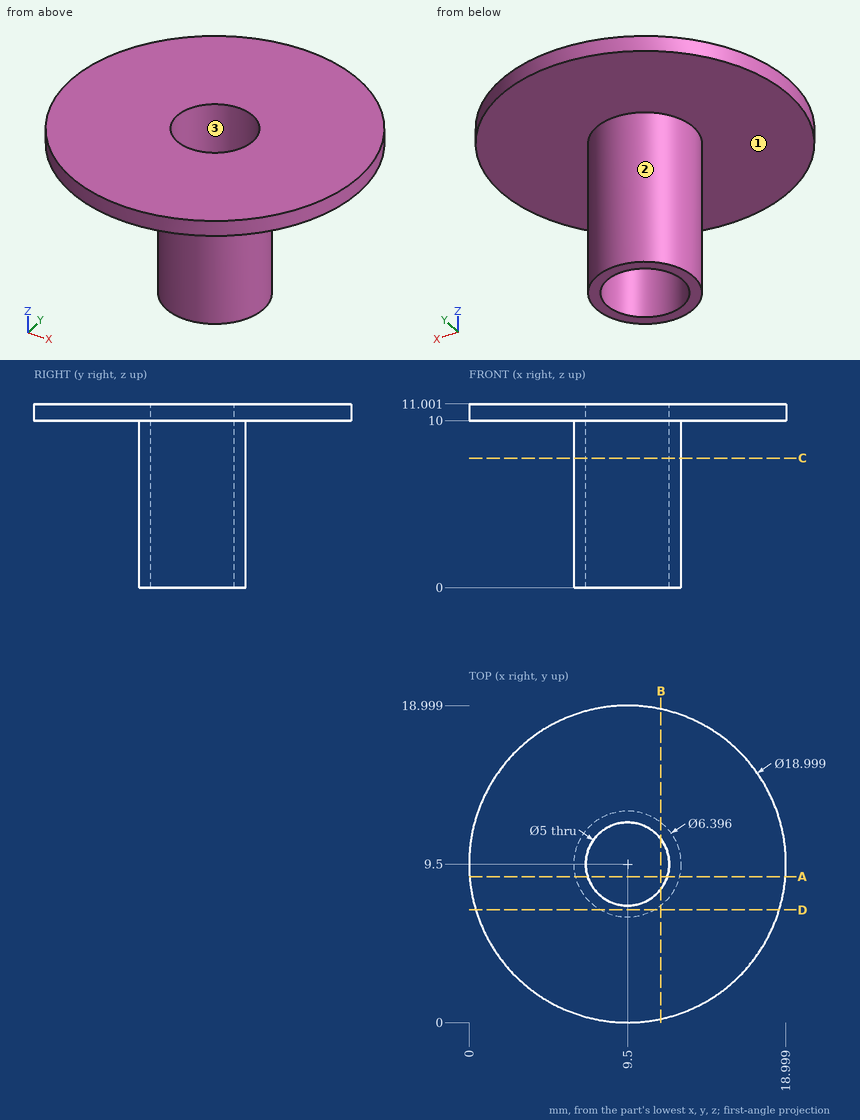
Verification items for this drawing (mm, ordinates from the low corner). Give positions to 0.01 mm unless a question says otherwise; leave off trailing zeros. Write each loop counter-clockwise with the first axis right and the second up, starting at its lowest first coordinate (ties: lowest second). Pieces come first, ordered by that corner, then holes. Notation, with made-up numbers: (53, 34) -> (57, 34) arc R20 ccw to (57, 42) -> close; hole circle Ø6 at (31.25, 39). An arc over 180 degrees is marked (long way). Use one line per item in the form item = value.
Item 1: Depth check by flat-ended pin: pin 1 Ø4 at (x, y) = (8.5, 11) entering from +Z; pin 2 Ø1 at (y, z) = (9, 4.5) entering from -X; pin 3 Ø3 at (y, z) = (17, 9) entering from -X (1 decimal); pin 4 Ø3 at (x, z) = (4, 7.5) entering from -Y. Enter the tip coordinate at first touch or a pass-through.
Results list:
pin_1 = 11
pin_2 = 6.3
pin_3 = 2.5
pin_4 = through
Item 2: Mould release check, pull along Y, two halves, no side actions. Record for the marked faces 1, 2 and 3: released by +Y, released by -Y, zero draft, split by the parting line, or undercut.
Results list:
face_1 = zero draft
face_2 = split by the parting line
face_3 = undercut
Item 3: Sectioned sample at B-B on x = 11.5. Enter the section's corners in (y, z) (1 decimal).
Results list:
outline = (0.2, 10) -> (7, 10) -> (7, 0) -> (8, 0) -> (8, 11) -> (0.2, 11) -> close; (11, 0) -> (12, 0) -> (12, 10) -> (18.8, 10) -> (18.8, 11) -> (11, 11) -> close
Item 4: Sectioned sample at C-C on z = 7.75. Enter the section's corners in (x, y) (1 decimal), plus the area to 3 significant figures.
Results list:
outline = circle Ø6.4 at (9.5, 9.5); hole circle Ø5 at (9.5, 9.5)
area = 12.5 mm2
Item 5: Sectioned sample at D-D on y = 6.75. Enter the section's corners in (x, z).
Results list:
outline = (0.41, 10) -> (7.87, 10) -> (7.87, 0) -> (11.13, 0) -> (11.13, 10) -> (18.59, 10) -> (18.59, 11) -> (0.41, 11) -> close
Item 6: Scan lines: line 1 (Y direction, x = 9.5, z = 6.5); line 2 (X direction, y = 9, z = 3.25); line 3 (Z direction, x = 2, y = 9.75). Record each from-to range of solid material in increasing order.
Results list:
line_1 = 6.3 to 7, 12 to 12.7
line_2 = 6.34 to 7.05, 11.95 to 12.66
line_3 = 10 to 11
Item 7: Sectioned sample at A-A on y = 8.75. Enter the section's corners in (x, z) (1 decimal).
Results list:
outline = (0, 10) -> (6.4, 10) -> (6.4, 0) -> (7.1, 0) -> (7.1, 11) -> (0, 11) -> close; (11.9, 0) -> (12.6, 0) -> (12.6, 10) -> (19, 10) -> (19, 11) -> (11.9, 11) -> close
